from build123d import *

# Parameters (mm, degrees)
F1_DEPTH = 4.7625
F3_D     = 6.35
F4_R     = 3.175
F5_DEPTH = 25.4


with BuildPart() as f1:
    # F0 (on Front) → F1 (new body, symmetric)
    with BuildSketch(Plane.XZ):
        with BuildLine():
            ThreePointArc((107.4907893633, -0.6147240541), (0, 107.4925471073), (-107.4907893633, -0.6147240541))
            Line((-107.4907893633, -0.6147240541), (107.4907893633, -0.6147240541))
        make_face()
    extrude(amount=F1_DEPTH, both=True)

    # F3 (through all)
    with Locations(Plane.XZ.offset(4.7625)):
        with Locations((23.8125, 18.4352759459), (87.3125, 18.6611738243), (47.9041955289, 77.1880736359), (23.5866021216, 81.9352759459), (68.5540466837, 63.4962904729), (82.392402939, 42.9443763274), (-23.8125, 18.4352759459), (-23.5866021216, 81.9352759459), (-47.9041955289, 77.1880736359), (-68.5540466837, 63.4962904729), (-82.392402939, 42.9443763274), (-87.3125, 18.6611738243)):
            Hole(F3_D / 2)

    # F4 (on face) → F5 (cut)
    with BuildSketch(Plane.XZ.offset(4.7625)):
        with BuildLine():
            Line((-135.8842252305, -8.5859880761), (4.7625, -8.5859880761))
            Line((4.7625, -8.5859880761), (4.7625, -0.6147240541))
            Line((4.7625, -0.6147240541), (-107.4907893633, -0.6147240541))
            ThreePointArc((-107.4907893633, -0.6147240541), (-74.5276330195, 77.4614717141), (4.7625, 107.3869930548))
            Line((4.7625, 107.3869930548), (4.7625, 118.4140119239))
            Line((4.7625, 118.4140119239), (-135.8842252305, 118.4140119239))
            Line((-135.8842252305, 118.4140119239), (-135.8842252305, -8.5859880761))
        make_face()
        with BuildLine():
            Line((-107.4907893633, -0.6147240541), (4.7625, -0.6147240541))
            Line((4.7625, -0.6147240541), (4.7625, 107.3869930548))
            ThreePointArc((4.7625, 107.3869930548), (-74.5276330195, 77.4614717141), (-107.4907893633, -0.6147240541))
        make_face()
        with Locations((-87.3125, 18.6611738243)):
            Circle(F4_R, mode=Mode.SUBTRACT)
        with Locations((-23.8125, 18.4352759459)):
            Circle(F4_R, mode=Mode.SUBTRACT)
        with Locations((-82.392402939, 42.9443763274)):
            Circle(F4_R, mode=Mode.SUBTRACT)
        with Locations((-68.5540466837, 63.4962904729)):
            Circle(F4_R, mode=Mode.SUBTRACT)
        with Locations((-47.9041955289, 77.1880736359)):
            Circle(F4_R, mode=Mode.SUBTRACT)
        with Locations((-23.5866021216, 81.9352759459)):
            Circle(F4_R, mode=Mode.SUBTRACT)
    extrude(amount=-F5_DEPTH, mode=Mode.SUBTRACT)


solid = f1.part
Design review of the part built by this model. Coordinates are the model's own, in mm. Round coordinates to 2 decimals unless told otherwise and drop trailing zeros. Write each loop counter-clockwise with the first axis right and the second up, starting at its lowest first coordinate (ties: lowest second). Pieces come first, ordered by that corner, then holes. Notation, with made-up numbers: (78, -29) - (131, -29) arc R23 cw to (131, -16) - close; hole circle Ø8 at (-12.5, -14). An arc over 180 degrees is marked (long way). Use a Markdown table: item, result. Add a question column.
1. Mouldability with a two-part tool opening along X and no side actions: class faces 1 (the face through (70.894, 0.067, 65.642)), 2 (the face through (78.68, -0.07, 73.24)), 3 (the face through (55, 0, -0.615)) as +X half, -X half, draft (parallel to the pull), parting line (faces both ways), or undercut.
2. Wall thickness on probe 1 along X at (y, z) = (1.5, 19); probe 2 along X at (y, z) = (3.5, 42.5); probe 3 along Z at (x, y) = (86.5, 1): over which ranges is each line inside the solid? List them lowest first.
3. We need section A-A (y = -0.5). Count the separate pieces of the cut face and the enclosed holes in it, then the cut area to 3 significant figures.
4. Clearance check with flat-ended pins moving along their axes: pin 1 (1.5 mm diameter, centred on y = -1.5, z = 91.5, fed in from +X); pin 2 (7.5 mm diameter, centred on x = 87.31, z = 18.66, fed in from +Y); pin 3 (4 mm diameter, centred on y = -1, z = 45, fed in from +X). State where each tip first meets the part, or that it passes through.
5. We need section C-C (x = 74). State the section outline as (y, z) points.
6. We need section B-B (z = 58). State the section outline as (x, y) points.
Output:
| question | item | result |
|---|---|---|
| 1 | face 1 | undercut |
| 1 | face 2 | +X half |
| 1 | face 3 | draft |
| 2 | probe 1 | x = 4.76 to 20.69, 26.94 to 84.16, 90.47 to 105.8 |
| 2 | probe 2 | x = 4.76 to 79.25, 85.54 to 98.73 |
| 2 | probe 3 | z = -0.61 to 15.59, 21.73 to 63.82 |
| 3 | separate pieces | 1 |
| 3 | enclosed holes | 6 |
| 3 | area | 8,440 mm2 |
| 4 | pin 1 | stops at x = 57.61 |
| 4 | pin 2 | stops at y = 4.76 |
| 4 | pin 3 | stops at x = 98.52 |
| 5 | outline | (-4.76, -0.61) - (4.76, -0.61) - (4.76, 77.97) - (-4.76, 77.97) - close |
| 6 | outline | (4.76, -4.76) - (90.5, -4.76) - (90.5, 4.76) - (4.76, 4.76) - close |
